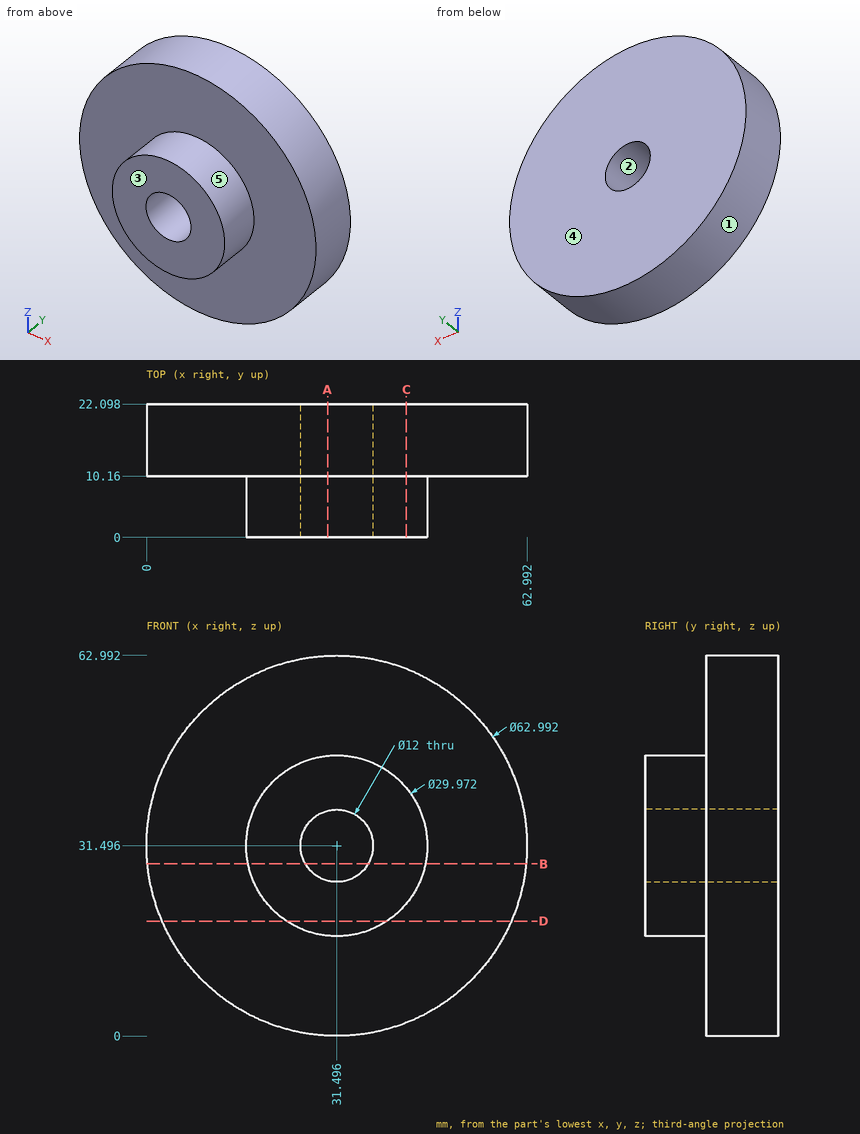
Part print with two shaded views. Sizes in mm from the minimum x, y, z corner. A direction names the side the tool comes from. Round coordinates to 2 decimals unless told otherwise and drop trailing zeros. Order: outer loops, then holes, each group sorted by start corner. A loop starts at its lowest first (then second) coordinate and runs counter-clockwise, first axis right, second up.
(1) Band-saw the part on C-C (x = 43). List the corners of the cut face in (y, z), then the cut area to 3 significant figures.
(2) Pin check, flat tips, straight feed: pin 1 (6 mm diameter, centred on y = 10.5, z = 56, fed in from +X); pin 2 (1 mm diameter, centred on y = 10.5, z = 24.5, fed in from -X); pin 3 (1 mm diameter, centred on y = 15, z = 37.5, fed in from +X); pin 4 (19 mm diameter, centred on x = 31.496, z = 31.496, fed in from -Y). Stop position of each tip, or through.
(3) Band-saw the part on A-A (x = 30). List the corners of the cut face in (y, z).
(4) 3-axis set-ups, long thin cutter, end or side, ignore diameter. For the marked faces 4 and 5: which of +Z, -Z, +X, -X, +Y, -Y reach the whole face in a straight line?
(5) Drill centre lines: line 1 (Y direction, x = 17.5, z = 16); line 2 (Z direction, x = 34, y = 8.25); line 3 (X direction, y = 20.75, z = 37). Where is each one in solid material? Low to high.
(6) Pull direction Z, two halves, no side cores. Call the marked faces 1, 2 and 3: released by +Z, released by -Z, zero draft, split by the parting line, or undercut.
(7) Band-saw the part on D-D (z = 19). List the corners of the cut face in (x, y), then the cut area to 3 significant figures.
(8) Band-saw the part on B-B (z = 28.5). List the corners of the cut face in (x, y), then the cut area to 3 significant figures.
Verdict:
1. outline: (0, 21.89) - (10.16, 21.89) - (10.16, 2.18) - (22.1, 2.18) - (22.1, 60.82) - (10.16, 60.82) - (10.16, 41.1) - (0, 41.1) - close
1. area: 895 mm2
2. pin 1: stops at x = 54.51
2. pin 2: stops at x = 0.68
2. pin 3: stops at x = 62.51
2. pin 4: stops at y = 0
3. outline: (0, 16.58) - (10.16, 16.58) - (10.16, 0.04) - (22.1, 0.04) - (22.1, 25.69) - (0, 25.69) - close; (0, 37.31) - (22.1, 37.31) - (22.1, 62.96) - (10.16, 62.96) - (10.16, 46.41) - (0, 46.41) - close
4. face 4: +Z, -Z, +X, -X, +Y
4. face 5: -Y
5. line 1: y = 10.16 to 22.1
5. line 2: z = 16.72 to 26.04, 36.95 to 46.27
5. line 3: x = 0.48 to 29.11, 33.88 to 62.51
6. face 1: split by the parting line
6. face 2: undercut
6. face 3: zero draft
7. outline: (2.58, 10.16) - (23.22, 10.16) - (23.22, 0) - (39.77, 0) - (39.77, 10.16) - (60.41, 10.16) - (60.41, 22.1) - (2.58, 22.1) - close
7. area: 858 mm2
8. outline: (0.14, 10.16) - (16.81, 10.16) - (16.81, 0) - (26.3, 0) - (26.3, 22.1) - (0.14, 22.1) - close; (36.69, 0) - (46.18, 0) - (46.18, 10.16) - (62.85, 10.16) - (62.85, 22.1) - (36.69, 22.1) - close
8. area: 817 mm2
